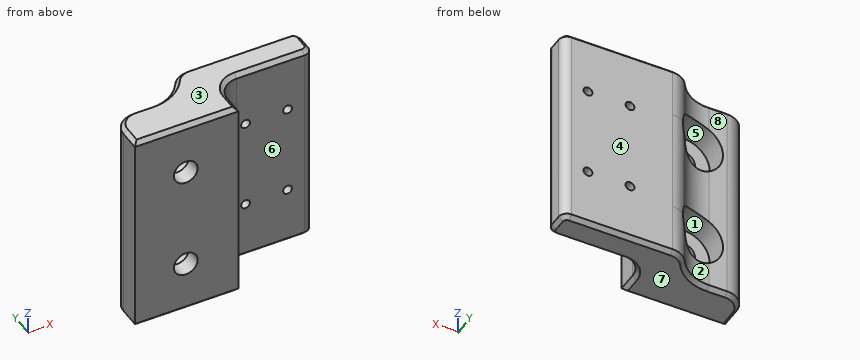
from build123d import *

# Parameters (mm, degrees)
BOSS_EXTRUDE1_DEPTH = 25.5
SKETCH3_R           = 2.921
CUT_EXTRUDE1_DEPTH  = 39.320882036
SKETCH3_4_R         = 6.5
SKETCH3_4_R_2       = 2.921
CUT_EXTRUDE2_DEPTH  = 6
SKETCH9_R           = 1.0922
CUT_EXTRUDE3_DEPTH  = 41.712283159
FILLET1_R           = 10
FILLET2_R           = 5
FILLET4_R           = 2
CHAMFER1_SIZE       = 1


with BuildPart() as part:
    # Sketch1 → Boss-Extrude1 (new, symmetric)
    with BuildSketch(Plane.XY):
        Polygon((-22.2, -8.5), (3.2, -8.5), (3.2, 1.5), (26.8, 1.5), (26.8, 8.5), (-3.2, 8.5), (-3.2, 1.5), (-22.2, 1.5), align=None)
    extrude(amount=BOSS_EXTRUDE1_DEPTH, both=True)

    # Sketch3 → Cut-Extrude1 (cut, through all)
    with BuildSketch(Plane(origin=(0, 1.5, 0), x_dir=(1, 0, 0), z_dir=(0, 1, 0))):
        with Locations(Location((-9.7, -12.7, 0), (0, 0, 180))):
            Circle(SKETCH3_R)
    cut_extrude1 = extrude(amount=-CUT_EXTRUDE1_DEPTH, mode=Mode.SUBTRACT)

    # Sketch3<4> → Cut-Extrude2 (cut)
    with BuildSketch(Plane(origin=(0, 1.5, 0), x_dir=(1, 0, 0), z_dir=(0, 1, 0))):
        with Locations(Location((-9.7, -12.7, 0), (0, 0, 180))):
            Circle(SKETCH3_4_R)
        with Locations(Location((-9.7, -12.7, 0), (0, 0, 180))):
            Circle(SKETCH3_4_R_2, mode=Mode.SUBTRACT)
    cut_extrude2 = extrude(amount=-CUT_EXTRUDE2_DEPTH, mode=Mode.SUBTRACT)

    # Mirror1: Cut-Extrude1, Cut-Extrude2 across plane
    add(cut_extrude1.mirror(Plane.XY), mode=Mode.SUBTRACT)
    add(cut_extrude2.mirror(Plane.XY), mode=Mode.SUBTRACT)

    # Sketch9 → Cut-Extrude3 (cut, through all)
    with BuildSketch(Plane(origin=(0, 8.5, 0), x_dir=(1, 0, 0), z_dir=(0, 1, 0))):
        with Locations(Location((10.4078, 11.1, 0), (0, 0, 180))):
            Circle(SKETCH9_R)
        with Locations(Location((20.7078, -11.1, 0), (0, 0, 180))):
            Circle(SKETCH9_R)
        with Locations(Location((20.7078, 11.1, 0), (0, 0, 180))):
            Circle(SKETCH9_R)
        with Locations(Location((10.4078, -11.1, 0), (0, 0, 180))):
            Circle(SKETCH9_R)
    extrude(amount=-CUT_EXTRUDE3_DEPTH, mode=Mode.SUBTRACT)

    # Fillet1
    # the kernel refuses this fillet: 10 mm, written as the material it adds along each edge
    with BuildSketch(Plane(origin=(-3.2, 1.5, 25.5), x_dir=(0, 1, 0), z_dir=(0, 0, -1))) as fillet1_piece_1_section:
        with BuildLine():
            CenterArc((10, -9.539392014), FILLET1_R, 107.457603124, 72.542396876)
            Line((0, -9.539392014), (0, 0))
            Line((0, 0), (7, 0))
        make_face()
    fillet1_piece_1 = extrude(amount=12.8, mode=Mode.PRIVATE)
    fillet1_piece_1 = fillet1_piece_1 - Plane(origin=(-9.7, 1.5, 12.7), x_dir=(-1, 0, 0), z_dir=(0, 1, 0)) * Cylinder(6.5, 64, mode=Mode.PRIVATE)
    add(fillet1_piece_1)
    with BuildSketch(Plane(origin=(-3.2, 1.5, -12.700000035), x_dir=(0, 1, 0), z_dir=(0, 0, -1))) as fillet1_piece_2_section:
        with BuildLine():
            CenterArc((10, -9.539392014), FILLET1_R, 107.457603124, 72.542396876)
            Line((0, -9.539392014), (0, 0))
            Line((0, 0), (7, 0))
        make_face()
    fillet1_piece_2 = extrude(amount=12.799999965, mode=Mode.PRIVATE)
    fillet1_piece_2 = fillet1_piece_2 - Plane(origin=(-9.7, 1.5, -12.7), x_dir=(-1, 0, 0), z_dir=(0, 1, 0)) * Cylinder(6.5, 64, mode=Mode.PRIVATE)
    add(fillet1_piece_2)
    with BuildSketch(Plane(origin=(-3.2, 1.5, 12.7), x_dir=(0, 1, 0), z_dir=(0, 0, -1))) as fillet1_piece_3_section:
        with BuildLine():
            CenterArc((10, -9.539392014), FILLET1_R, 107.457603124, 72.542396876)
            Line((0, -9.539392014), (0, 0))
            Line((0, 0), (7, 0))
        make_face()
    fillet1_piece_3 = extrude(amount=25.400000035, mode=Mode.PRIVATE)
    fillet1_piece_3 = fillet1_piece_3 - Plane(origin=(-9.7, 1.5, -12.7), x_dir=(-1, 0, 0), z_dir=(0, 1, 0)) * Cylinder(6.5, 89, mode=Mode.PRIVATE)
    fillet1_piece_3 = fillet1_piece_3 - Plane(origin=(-9.7, 1.5, 12.7), x_dir=(-1, 0, 0), z_dir=(0, 1, 0)) * Cylinder(6.5, 89, mode=Mode.PRIVATE)
    add(fillet1_piece_3)

    # Fillet2
    # the kernel refuses this fillet: 5 mm, written as the material it adds along each edge
    with BuildSketch(Plane(origin=(3.2, 1.5, -25.5), x_dir=(0, -1, 0), z_dir=(0, 0, 1))) as fillet2_piece_1:
        with BuildLine():
            CenterArc((FILLET2_R, FILLET2_R), FILLET2_R, 180, 90)
            Line((0, FILLET2_R), (0, 0))
            Line((0, 0), (FILLET2_R, 0))
        make_face()
    extrude(amount=51)
    # the kernel refuses this fillet: 5 mm, written as the material it takes off along each edge
    with BuildSketch(Plane(origin=(-3.2, 8.5, -33.372963816), x_dir=(1, 0, 0), z_dir=(0, 0, 1))) as fillet2_2_piece_1:
        with BuildLine():
            CenterArc((3.149185526, -5), FILLET2_R, 90, 57.769047364)
            ThreePointArc((-1.080340321, -2.333333333), (-0.464861443, -1.201534828), (0, 0))
            Line((0, 0), (3.149185526, 0))
        make_face()
    extrude(amount=20.67296378, mode=Mode.SUBTRACT)
    with BuildSketch(Plane(origin=(-22.2, 1.5, 38), x_dir=(1, 0, 0), z_dir=(0, 0, -1))) as fillet2_2_piece_2:
        with BuildLine():
            CenterArc((FILLET2_R, FILLET2_R), FILLET2_R, 180, 90)
            Line((0, FILLET2_R), (0, 0))
            Line((0, 0), (FILLET2_R, 0))
        make_face()
    extrude(amount=76, mode=Mode.SUBTRACT)
    with BuildSketch(Plane(origin=(-3.2, 8.5, -12.700000035), x_dir=(-0.42015348282673015, -0.9074530571156663, 0), z_dir=(0, 0, 1))) as fillet2_2_piece_3:
        with BuildLine():
            CenterArc((3.214124019, 4.958505447), FILLET2_R, 204.84427788, 57.769047364)
            Line((-1.323141267, 2.857738033), (0, 0))
            ThreePointArc((0, 0), (1.285649607, 0.082989105), (2.571299215, 0))
        make_face()
    extrude(amount=25.400000035, mode=Mode.SUBTRACT)
    with BuildSketch(Plane(origin=(-3.2, 8.5, 12.7), x_dir=(1, 0, 0), z_dir=(0, 0, 1))) as fillet2_2_piece_4:
        with BuildLine():
            CenterArc((3.149185526, -5), FILLET2_R, 90, 57.769047364)
            ThreePointArc((-1.080340321, -2.333333333), (-0.464861443, -1.201534828), (0, 0))
            Line((0, 0), (3.149185526, 0))
        make_face()
    extrude(amount=20.672963816, mode=Mode.SUBTRACT)

    # Fillet4
    fillet4_edges = [part.edges().sort_by_distance(p)[0] for p in [
        (26.8, 8.5, 0),
        (26.8, 1.5, 0),
    ]]
    fillet(fillet4_edges, radius=FILLET4_R)

    # Chamfer1
    chamfer1_edges = [part.edges().sort_by_distance(p)[0] for p in [
        (3.2, -6, -25.5),
        (12.374592763, 8.5, 25.5),
        (-9.5, -8.5, -25.5),
        (12.374592763, 8.5, -25.5),
        (26.8, 5, -25.5),
        (26.214213562, 2.085786438, -25.5),
        (26.214213562, 7.914213562, -25.5),
        (26.8, 5, 25.5),
        (26.214213562, 2.085786438, 25.5),
        (26.214213562, 7.914213562, 25.5),
        (3.2, -6, 25.5),
        (-14.969696007, 1.5, -25.5),
        (-14.969696007, 1.5, 25.5),
        (-7.908933099, 2.744049642, -25.5),
        (-7.908933099, 2.744049642, 25.5),
        (-22.2, -6, 25.5),
        (16.5, 1.5, 25.5),
        (-20.735533906, 0.035533906, 25.5),
        (-2.466043931, 7.877975179, 25.5),
        (-22.2, -6, -25.5),
        (-9.5, -8.5, 25.5),
        (16.5, 1.5, -25.5),
        (-20.735533906, 0.035533906, -25.5),
        (-2.466043931, 7.877975179, -25.5),
        (4.664466094, 0.035533906, -25.5),
        (4.664466094, 0.035533906, 25.5),
    ]]
    chamfer(chamfer1_edges, length=CHAMFER1_SIZE)


solid = part.part
Part model, mm, in its own coordinate system. Face numbers are marked on the shaded views. A direction names the side the tool comes from. Round coordinates to 2 decimals unless told otherwise and drop trailing zeros. Loops run counter-clockwise (first coordinate to the right, second up) from the corner with the lowest first, then second, coordinate; pieces in that order, holes last. Notation, with made-up numbers: (22.5, 23) - (28.5, 23) arc R20 cw to (28.5, 33) - close; hole circle Ø2 at (48.5, -33). An arc over 180 degrees is marked (long way). Answer as a JSON object with one key per item and string values.
Item 1: Tool access for the marked faces 4, 5, 6, 7 and 8: list every direction of +Z, -Z, +X, -X, +Y, -Y with a clear straight run to the whole face (end or side of a thin tool).
Output:
{"face 4": "+Z, -Z, +X, -X, +Y", "face 5": "+Y", "face 6": "+Z, -Z, +X, -Y", "face 7": "-Z, +X, -X, +Y, -Y", "face 8": "+Z, -Z, -X, +Y"}
Item 2: Pin check, flat tips, straight feed: pin 1 (3.5 mm diameter, centred on x = -9.7, z = 12.7, fed in from -Y); pin 2 (1 mm diameter, centred on y = 4.5, z = -14, fed in from -X); pin 3 (4 mm diameter, centred on x = -9, z = -13.5, fed in from +Y); pin 4 (10.5 mm diameter, centred on x = -9.7, z = -12.7, fed in from -Y). Stop position of each tip, or through.
Output:
{"pin 1": "through", "pin 2": "x = -3.45", "pin 3": "y = -4.5", "pin 4": "y = -8.5"}
Item 3: Band-saw the part on D-D on z = 14. List the corners of the cut face in (x, y), plus the area to 3 significant figures.
Output:
{"outline": "(-22.2, -8.5) - (-12.32, -8.5) - (-12.32, -4.5) - (-16.07, -4.5) - (-16.07, 1.5) - (-17.2, 1.5) arc R5 ccw to (-22.2, -3.5) - close; (-7.08, -8.5) - (3.2, -8.5) - (3.2, -3.5) arc R5 cw to (8.2, 1.5) - (24.8, 1.5) arc R2 ccw to (26.8, 3.5) - (26.8, 6.5) arc R2 ccw to (24.8, 8.5) - (-0.05, 8.5) arc R5 ccw to (-3.33, 7.27) - (-3.33, -4.5) - (-7.08, -4.5) - close", "area": "365 mm2"}
Item 4: Wall check: L1, parallel to Z at x = -11, y = -1.5; L2, parallel to Z at x = -13, y = 0; L3, parallel to X at y = -6.4, z = -12.7. Give the ranges that are in metal, low to high.
Output:
{"L1": "-25.5 to -19.07, -6.33 to 6.33, 19.07 to 25.5", "L2": "-25.5 to -18.3, -7.1 to 7.1, 18.3 to 25.5", "L3": "-22.2 to -12.62, -6.78 to 3.2"}
Item 5: Pull direction X, two halves, no side cores. Call the marked faces 1, 2 and 3: pulls with the +X half, pulls with the -X half, needs draft (parallel to the pull), parting line crosses it, or undercut.
Output:
{"face 1": "undercut", "face 2": "pulls with the -X half", "face 3": "needs draft"}
Item 6: Band-saw the part on A-A on z = -1. List the corners of the cut face in (x, y).
Output:
{"outline": "(-22.2, -8.5) - (3.2, -8.5) - (3.2, -3.5) arc R5 cw to (8.2, 1.5) - (24.8, 1.5) arc R2 ccw to (26.8, 3.5) - (26.8, 6.5) arc R2 ccw to (24.8, 8.5) - (-0.05, 8.5) arc R5 ccw to (-4.28, 6.17) arc R10 cw to (-12.74, 1.5) - (-17.2, 1.5) arc R5 ccw to (-22.2, -3.5) - close"}
Item 7: Band-saw the part on B-B on y = -5.75. List the corners of the cut face in (x, z).
Output:
{"outline": "(-22.2, -24.5) - (-21.2, -25.5) - (2.2, -25.5) - (3.2, -24.5) - (3.2, 24.5) - (2.2, 25.5) - (-21.2, 25.5) - (-22.2, 24.5) - close; hole circle Ø5.84 at (-9.7, -12.7); hole circle Ø5.84 at (-9.7, 12.7)"}
Item 8: Band-saw the part on C-C on x = 21. List the corners of the cut face in (y, z).
Output:
{"outline": "(1.5, -24.5) - (2.5, -25.5) - (7.5, -25.5) - (8.5, -24.5) - (8.5, -12.15) - (1.5, -12.15) - close; (1.5, -10.05) - (8.5, -10.05) - (8.5, 10.05) - (1.5, 10.05) - close; (1.5, 12.15) - (8.5, 12.15) - (8.5, 24.5) - (7.5, 25.5) - (2.5, 25.5) - (1.5, 24.5) - close"}
